```python
from build123d import *

# Parameters (mm, degrees)
F1_DEPTH = 30
F2_DEPTH = 60
F3_DEPTH = 15
F4_R     = 5
F5_SIZE  = 5
F6_R     = 5


with BuildPart() as f1:
    # F0 (on Front) → F1 (new body, symmetric)
    with BuildSketch(Plane.XZ):
        with BuildLine():
            Line((17.5, 20), (37.5, 20))
            Line((37.5, 20), (37.5, 30))
            ThreePointArc((37.5, 30), (40.428932, 37.071068), (47.5, 40))
            Line((47.5, 40), (74.281626, 40))
            Line((74.281626, 40), (74.281626, 60))
            Line((74.281626, 60), (59.462495, 60))
            Line((59.462495, 60), (47.5, 60))
            ThreePointArc((47.5, 60), (26.286797, 51.213203), (17.5, 30))
            Line((17.5, 30), (17.5, 20))
        make_face()
        Polygon((74.281626, 70), (74.281626, 60), (74.281626, 40), (74.281626, 30), (114.281626, 30), (114.281626, 70), align=None)
    extrude(amount=F1_DEPTH, both=True)

    # F0 (on Front) → F2 (join, symmetric)
    with BuildSketch(Plane.XZ):
        Polygon((-37.5, -20), (37.5, -20), (37.5, 20), (17.5, 20), (-37.5, 20), align=None)
    extrude(amount=F2_DEPTH, both=True)

    # F0 (on Front) → F3 (join, symmetric)
    with BuildSketch(Plane.XZ):
        with BuildLine():
            add(Edge.make_bspline(
                [(-37.5, 20), (-19.089822, 55.62811), (19.591885, 66.455275), (59.462495, 60)],
                knots=[0, 0, 0, 0, 104.88911, 104.88911, 104.88911, 104.88911], degree=3))
            Line((-37.5, 20), (17.5, 20))
            Line((17.5, 20), (17.5, 30))
            ThreePointArc((17.5, 30), (26.286797, 51.213203), (47.5, 60))
            Line((47.5, 60), (59.462495, 60))
        make_face()
    extrude(amount=F3_DEPTH, both=True)

    # F4
    f4_edges = [f1.edges().sort_by_distance(p)[0] for p in [
        (0, -60, 20),
        (-37.5, -60, 0),
        (0, -60, -20),
        (37.5, -60, 0),
    ]]
    fillet(f4_edges, radius=F4_R)

    # F5
    f5_edges = [f1.edges().sort_by_distance(p)[0] for p in [
        (74.281626, 0, 70),
        (74.281626, 0, 30),
    ]]
    chamfer(f5_edges, length=F5_SIZE)

    # F6
    f6_edges = [f1.edges().sort_by_distance(p)[0] for p in [
        (0, 60, 20),
        (-37.5, 60, 0),
        (0, 60, -20),
        (37.5, 60, 0),
    ]]
    fillet(f6_edges, radius=F6_R)


solid = f1.part
```
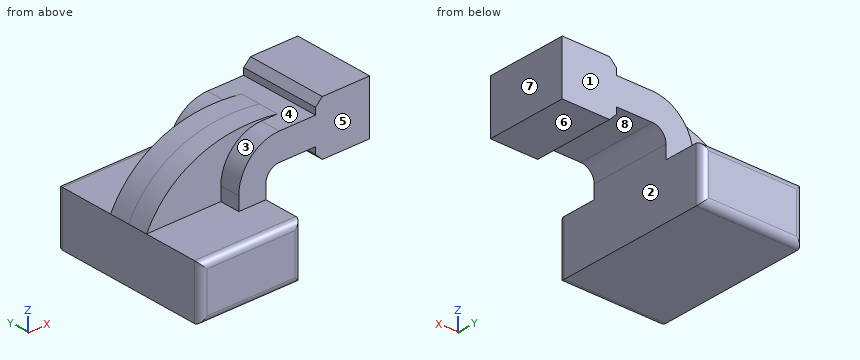
CAD build for the part. Positions are in the model's coordinates, mm. Face numbers are marked on the shaded views. A direction names the side the tool comes from. Round coordinates to 2 decimals unless told otherwise and drop trailing zeros. Write each loop counter-clockwise with the first axis right and the second up, starting at its lowest first coordinate (ties: lowest second). Pieces come first, ordered by that corner, then holes. Notation, with made-up numbers: (-5, -21.5) -> (7, -21.5) arc R23 ccw to (7, 3.5) -> close; hole circle Ø5 at (33, 41.25). An arc over 180 degrees is marked (long way). Answer in a Markdown table with one row per item. Add a question column.
Item 1: Which spindle directions (+Z, -Z, +X, -X, +Y, -Y) get a long thin tool onto all of the face, cutting with end or side? Do the marked faces 1, 2, 3, 4 and 5. Say none if no direction does.
Item 2: Drill centre lines: line 1 (X direction, y = 2.5, z = 20); line 2 (Y direction, x = -15, z = 37); line 3 (Z direction, x = 12, y = 29). Where is each one in solid material? Low to high. Write a range as from..to.
Item 3: Drop flat-ended pins along their axis: pin 1 Ø1.5 at (x, y) = (67.5, -30.5) entering from -Z; pin 2 Ø8 at (x, y) = (19, -18.5) entering from +Z; pin 3 Ø1 at (x, y) = (40.5, -18) entering from +Z. Give the stop position or say it passes through.
Item 4: Saw through at C-C, the plane x = 69. Write the cut outline in (y, z), then the cut area to 3 significant figures.
Item 5: Saw through at B-B, the plane z = -2. Write the cut outline in (x, y).
Item 6: Saw through at A-A, the plane y = 25.5. Write the cut outline in (x, z), then the cut area to 3 significant figures.
Item 7: Saw through at D-D, the plane y = -35. Write the cut outline in (x, z).
Item 8: Mould opens along X. For the marked faces 6, 7 and 8 say: pulls with the +X half, pulls with the -X half, needs draft (parallel to the pull), parting line crosses it, or undercut.
Findings below:
| question | item | result |
|---|---|---|
| 1 | face 1 | +Z, +X, -X, +Y |
| 1 | face 2 | -Z, +X, +Y, -Y |
| 1 | face 3 | +Z, -X, -Y |
| 1 | face 4 | +Z |
| 1 | face 5 | +Z, +X, -X, -Y |
| 2 | line 1 | x = -37.5..37.5 |
| 2 | line 2 | y = -15..15 |
| 2 | line 3 | z = -20..20 |
| 3 | pin 1 | stops at z = 40 |
| 3 | pin 2 | stops at z = 60.45 |
| 3 | pin 3 | stops at z = 59.29 |
| 4 | outline | (-30, 40) -> (30, 40) -> (30, 60) -> (-30, 60) -> close |
| 4 | area | 1,200 mm^2 |
| 5 | outline | (-37.5, -55) arc R5 ccw to (-32.5, -60) -> (32.5, -60) arc R5 ccw to (37.5, -55) -> (37.5, 55) arc R5 ccw to (32.5, 60) -> (-32.5, 60) arc R5 ccw to (-37.5, 55) -> close |
| 6 | outline | (-37.5, -20) -> (37.5, -20) -> (37.5, 30) arc R10 cw to (47.5, 40) -> (74.28, 40) -> (74.28, 35) -> (79.28, 30) -> (114.28, 30) -> (114.28, 70) -> (79.28, 70) -> (74.28, 65) -> (74.28, 60) -> (47.5, 60) arc R30 ccw to (17.5, 30) -> (17.5, 20) -> (-37.5, 20) -> close |
| 6 | area | 5,940 mm^2 |
| 7 | outline | (-37.5, -20) -> (37.5, -20) -> (37.5, 20) -> (-37.5, 20) -> close |
| 8 | face 6 | needs draft |
| 8 | face 7 | pulls with the +X half |
| 8 | face 8 | undercut |
